Read the model definition and answer for the solid it produces. Units are mm, in the model's axes. A direction names the side the tool comes from. Round coordinates to 2 decimals unless told otherwise and drop trailing zeros. Write each loop counter-clockwise with the first axis right and the second up, starting at its lowest first coordinate (ties: lowest second). Pieces come first, ordered by that corner, then holes. Notation, with made-up numbers: (7, -25.75) - (50, -25.75) arc R33 cw to (50, 8.25) - close; hole circle Ø6 at (65, 71). An arc over 180 degrees is marked (long way). Answer as CSV lines item,"result". Start each with the question number.
1) Find section B-B on y = 1. Determine the outline of the cut face in (x, z), then the cut area to 3 significant figures.
2) For a pull along Z with two mould halves and no side action, classify faces 1 (the flat face through (-2, 4, 65)), 2 (the flat face through (-17, 8, 38)), 3 (the flat face through (-45, 5, 38)), 4 (the conical face through (8.102, 9.861, 83.034)) as +Z half, -Z half, draft (parallel to the pull), parting line (faces both ways), or undercut.
3) Find section C-C on z = 73. Determine the outline of the cut face in (x, y), then the cut area to 3 significant figures.
4) Which of the six approach directions +Z, -Z, +X, -X, +Y, -Y give full straight-line access (tool end or side, diameter ignored) to faces 5 (the flat face through (1, 0, 38)), 6 (the flat face through (0, 4, 33))?
5) Consider line 1 along X through (y, z) = (1.5, 24); line 2 along Z through (x, y) = (-17, 5.75); line 3 along Y through (x, z) = (-32, 27.5). Determine where each line is inside the solid, lowest interval first.
6) This flat-tipped pin is pushed along its axis until it touches: pin 1 (1 mm diameter, centred on x = -34, z = -0.5, fed in from -Y). Where does it stop, or does it pass through?
7) Find section A-A on x = -16. Determine the outline of the cut face in (y, z).
Autodesk Inventor part; units mm, degrees
ref_plane "YZ Plane" through (0, 0, 0) normal (1, 0, 0) x (0, 1, 0)
ref_plane "XZ Plane" through (0, 0, 0) normal (0, 1, 0) x (-1, 0, 0)
ref_plane "XY Plane" through (0, 0, 0) normal (0, 0, 1) x (1, 0, 0)
sketch "Sketch1" plane through (0, 0, 0) normal (0, 1, 0) x (-1, 0, 0)
  line L0 (0, 0) -> (35, 0)
  line L1 (35, 0) -> (35, 75)
  line L2 (35, 75) -> (0, 75)
  line L3 (0, 75) -> (0, 0)
  line L4 (45, -10) -> (-10, -10)
  line L5 (-10, -10) -> (-10, 85)
  line L6 (-10, 85) -> (45, 85)
  line L7 (45, 85) -> (45, -10)
  line L8 (35, 0) -> (45, -10) construction
  arc A0 (40, -10) -> (45, -5) centre (40, -5) ccw
  line L9 (45, 37.5) -> (48.3975, 37.5) construction
  line L10 (17.5, 85) -> (17.5, 95.7522) construction
  arc A1 (45, 80) -> (40, 85) centre (40, 80) ccw
  arc A2 (-10, -5) -> (-5, -10) centre (-5, -5) ccw
  arc A3 (-5, 85) -> (-10, 80) centre (-5, 80) ccw
  line L11 (32, 75) -> (32, 65)
  line L12 (32, 65) -> (35, 65)
  line L13 (3, 75) -> (3, 65)
  line L14 (3, 65) -> (0, 65)
  dimension "d0" = 35
  dimension "d1" = 75
  dimension "d2" = 10
  dimension "d8" = 10
  dimension "d9" = 3
extrude "Extrusion1" add sketch "Sketch1" along normal blind 10 contours L3 L14 L13 L2 L11 L12 L1 L0 | L3 L2 L13 L14 | L12 L11 L2 L1 | L4 A2 L5 A3 L6 A1 L7 A0
extrude "Extrusion2" cut sketch "Sketch1" along normal blind 8 contours L3 L14 L13 L2 L11 L12 L1 L0
sketch "Sketch3" plane through (5, 0, -10) normal (0, 0, -1) x (-1, 0, 0)
  line L0 (45, 10) -> (0, 10)
  line L1 (22.5, 10) -> (22.5, 15.0736) construction
  line L2 (27.5, 8) -> (17.5, 8)
  line L3 (0, 10) -> (45, 10)
  line L4 (14.5, 5) -> (14.5, -4.5377)
  line L5 (30.5, -4.5377) -> (30.5, 5)
  line L6 (37, 0) -> (8, 0)
  line L7 (30.5, 0) -> (14.5, 0)
  arc A0 (30.5, 5) -> (27.5, 8) centre (27.5, 5) ccw
  arc A1 (17.5, 8) -> (14.5, 5) centre (17.5, 5) ccw
  line L8 (8, 8) -> (37, 8)
  point P0 (5, 0)
  point P1 (30.5, 8)
  point P2 (14.5, 8)
  dimension "d15" = 8
  dimension "d16" = 8
  dimension "d19" = 3
extrude "Extrusion3" [suppressed]
chamfer "Chamfer1" [suppressed]
chamfer "Chamfer2" distance 0.8 angle 45 8 edges at (-17.5, 10, -10) (-43.5355, 10, -8.5355) (-45, 10, 37.5) (-43.5355, 10, 83.5355) (-17.5, 10, 85) (8.5355, 10, 83.5355) (10, 10, 37.5) (8.5355, 10, -8.5355)
equation "\"d16\" = d15"
properties part number "scatola_sopra"
Check values:
1,outline,"(-45, -5) arc R5 ccw to (-40, -10) - (5, -10) arc R5 ccw to (10, -5) - (10, 80) arc R5 ccw to (5, 85) - (-40, 85) arc R5 ccw to (-45, 80) - close; hole (-35, 0) - (0, 0) - (0, 65) - (-3, 65) - (-3, 75) - (-32, 75) - (-32, 65) - (-35, 65) - close"
1,area,"2,640 mm^2"
2,face 1,"undercut"
2,face 2,"undercut"
2,face 3,"draft"
2,face 4,"+Z half"
3,outline,"(-45, 0) - (-32, 0) - (-32, 8) - (-3, 8) - (-3, 0) - (10, 0) - (10, 9.2) - (9.2, 10) - (-44.2, 10) - (-45, 9.2) - close"
3,area,"317 mm^2"
4,face 5,"+Z, -Z, +X, -X, -Y"
4,face 6,"-Y"
5,line 1,"x = -45 to -35, 0 to 10"
5,line 2,"z = -10 to 0, 75 to 85"
5,line 3,"y = 8 to 10"
6,pin 1,"stops at y = 0"
7,outline,"(0, -10) - (9.2, -10) - (10, -9.2) - (10, 84.2) - (9.2, 85) - (0, 85) - (0, 75) - (8, 75) - (8, 0) - (0, 0) - close"
